The model under review builds one solid part; all positions refer to its coordinate system, in mm. Give positions to 0.01 mm unless a question says otherwise; leave off trailing zeros. Order: outer loops, then holes, each group sorted by start corner. A loop starts at its lowest first (then second) coordinate and runs counter-clockwise, first axis right, second up. Notation, with made-up numbers: M -20.75,41.5 L 35.25,41.5 A30 ccw 35.25,66.5 Z; hole C 4.25,-1 d11. An arc over 180 degrees is marked long. One line per question, with ' | ' between items. Start each with the question number.
1. We need section B-B on y = 43. Write out the cut boundary in (x, z), then the cut area to 3 significant figures.
2. Wall thickness on L1, parallel to Y at x = -7.5, z = 1.15; L2, parallel to Y at x = 6, z = 2.6; L3, parallel to Y at x = -10.75, z = 0.9: over which ranges is each line inside the solid? List them lowest first.
3. We need section C-C on z = 1.6. Write out the cut boundary in (x, y).
4. We need section A-A on x = -7.5. Write out the cut boundary in (y, z), then the cut area to 3 significant figures.
5. The part is to be moulded in two halves that separate along Y. For faces 1 (the face through (7.734, -40.215, 1.479)), 2 (the face through (11.285, -47.465, 1.479)), 3 (the face through (0, 1, 0)), say which applies: +Y half, -Y half, draft (parallel to the pull), parting line (faces both ways), or undercut.
6. We need section D-D on x = -12. Write out the cut boundary in (y, z).
```python
from build123d import *

# Parameters (mm, degrees)
SKETCH1_W                = 27.5
SKETCH1_H                = 100
BOSS_EXTRUDE1_DEPTH      = 3
M3_CLEARANCE_HOLE1_D     = 3.6
M3_CLEARANCE_HOLE1_DEPTH = 30
M3_CLEARANCE_HOLE1_TIP   = 1.081549114
CHAMFER1_SIZE            = 5


with BuildPart() as part:
    # Sketch1 → Boss-Extrude1 (new body)
    with BuildSketch(Plane.XY):
        Rectangle(SKETCH1_W, SKETCH1_H)
    extrude(amount=BOSS_EXTRUDE1_DEPTH)

    # M3 Clearance Hole1
    with Locations(Plane.XY.offset(3)):
        with Locations((-7.5, 43), (7.5, 43), (7.5, 28), (-7.5, 28), (-7.5, -42), (7.5, -42)):
            Hole(M3_CLEARANCE_HOLE1_D / 2, depth=M3_CLEARANCE_HOLE1_DEPTH)
            with Locations((0, 0, -(M3_CLEARANCE_HOLE1_DEPTH + M3_CLEARANCE_HOLE1_TIP / 2))):  # 118° drill point
                Cone(0, M3_CLEARANCE_HOLE1_D / 2, M3_CLEARANCE_HOLE1_TIP, mode=Mode.SUBTRACT)

    # Chamfer1
    chamfer1_edges = [part.edges().sort_by_distance(p)[0] for p in [
        (13.75, -50, 1.5),
        (-13.75, -50, 1.5),
    ]]
    chamfer(chamfer1_edges, length=CHAMFER1_SIZE)


solid = part.part
```
Entries:
1) outline: M -13.75,0 L -9.3,0 L -9.3,3 L -13.75,3 Z; M -5.7,0 L 5.7,0 L 5.7,3 L -5.7,3 Z; M 9.3,0 L 13.75,0 L 13.75,3 L 9.3,3 Z | area: 60.9 mm^2
2) L1: y = -50 to -43.8, -40.2 to 26.2, 29.8 to 41.2, 44.8 to 50 | L2: y = -50 to -42.99, -41.01 to 27.01, 28.99 to 42.01, 43.99 to 50 | L3: y = -48 to 50
3) outline: M -13.75,-45 L -8.75,-50 L 8.75,-50 L 13.75,-45 L 13.75,50 L -13.75,50 Z; hole C -7.5,-42 d3.6; hole C -7.5,28 d3.6; hole C -7.5,43 d3.6; hole C 7.5,-42 d3.6; hole C 7.5,28 d3.6; hole C 7.5,43 d3.6
4) outline: M -50,0 L -43.8,0 L -43.8,3 L -50,3 Z; M -40.2,0 L 26.2,0 L 26.2,3 L -40.2,3 Z; M 29.8,0 L 41.2,0 L 41.2,3 L 29.8,3 Z; M 44.8,0 L 50,0 L 50,3 L 44.8,3 Z | area: 268 mm^2
5) face 1: undercut | face 2: -Y half | face 3: draft
6) outline: M -46.75,0 L 50,0 L 50,3 L -46.75,3 Z
